For this review, take the finished solid that the model builds, in its own axes (mm). A direction names the side the tool comes from. Round coordinates to 2 decimals unless told otherwise and drop trailing zeros. Order: outer loops, then holes, each group sorted by start corner. A loop starts at its lowest first (then second) coordinate and runs counter-clockwise, first axis right, second up. Notation, with made-up numbers: (-20.5, -38) - (23.5, -38) arc R27 ccw to (23.5, -19) - close; hole circle Ø7 at (25, 51.25). An arc over 180 degrees is marked (long way). Write each question's results on one line, items separated by ' | '. Start each with the question number.
(1) For faces 1 (the flat face through (-19.35, -1.5, -6.77)), 2 (the flat face through (-20.227, -1.503, 43.929)), list the 3-axis set-ups (+Z, -Z, +X, -X, +Y, -Y) from which the entire face can be reached by the end or side of a thin tool; tool diameter is ignored.
(2) Take a section at B-B, the plane x = -4. Give the boundary of the cut face in (y, z), plus the area to 3 significant figures.
(3) For L1, parallel to X at y = -0.75, z = -46; L2, parallel to X at y = -2.05, z = 55.5; L3, parallel to X at y = -1.15, z = 69.5, list the stretches that pass through material, from the lowest coordinate up. Write a range as from..to.
(4) Take a section at A-A, the plane y = -1. Give the number of separate pieces and of enclosed holes in the cut face, plus the area to 3 significant figures.
(5) Take a section at C-C, the plane z = 37. Give the boundary of the cut face in (x, y).
(6) Draft analysis for pull direction Z (two halves, no side actions). For faces 3 (the flat face through (-45.517, -1.503, -15.58)), 4 (the flat face through (-30, 0, -3)), 5 (the cylindrical face through (-35.836, -1.503, -48.481)), state which applies: pulls with the +Z half, pulls with the -Z half, needs draft (parallel to the pull), parting line crosses it, or undercut.
(7) Insertion check: pin 1 Ø10 at (x, z) = (-38, 17) entering from +Y; pin 2 Ø1.5 at (y, z) = (-1.5, 2) entering from -X; pin 3 Ø6 at (x, z) = (-32.87, 17.29) entering from -Y. Each pin has a flat end and moves straight along its axis. Give the tip position at first contact, or say it passes through.
```python
from build123d import *

# Parameters (mm, degrees)
F0_R     = 3.175
F0_R_2   = 2.8967213822
F0_R_3   = 4.9231792558
F0_R_4   = 3.7359067091
F0_R_5   = 3.1164885501
F1_DEPTH = 3.048


with BuildPart() as f1:
    # F0 (on Front) → F1 (new body)
    with BuildSketch(Plane.XZ):
        with BuildLine():
            ThreePointArc((-42.3213338093, 69.2824711493), (-33.4675240871, 58.5855412551), (-23.3460408451, 68.0918461493))
            ThreePointArc((-23.3460408451, 68.0918461493), (-23.3647359509, 68.6883293913), (-23.4207478809, 69.2824711493))
            ThreePointArc((-23.4207478809, 69.2824711493), (-32.8710408451, 77.6168461493), (-42.3213338093, 69.2824711493))
        make_face()
        with Locations((-32.8710408451, 68.0918461493)):
            Circle(F0_R, mode=Mode.SUBTRACT)
        with BuildLine():
            ThreePointArc((-23.4207478809, 69.2824711493), (-23.3647359509, 68.6883293913), (-23.3460408451, 68.0918461493))
            ThreePointArc((-23.3460408451, 68.0918461493), (-33.4675240871, 58.5855412551), (-42.3213338093, 69.2824711493))
            Line((-42.3213338093, 69.2824711493), (-48.6215291188, 19.2762211493))
            ThreePointArc((-48.6215291188, 19.2762211493), (-32.8710408451, 33.1668461493), (-17.1205525714, 19.2762211493))
            Line((-17.1205525714, 19.2762211493), (-23.4207478809, 69.2824711493))
        make_face()
        with Locations((-36.0460408451, 53.8170461493)):
            Circle(F0_R_2, mode=Mode.SUBTRACT)
        with BuildLine():
            ThreePointArc((-16.9960408451, 17.2918461493), (-17.0271993547, 18.2859848859), (-17.1205525714, 19.2762211493))
            ThreePointArc((-17.1205525714, 19.2762211493), (-32.8710408451, 33.1668461493), (-48.6215291188, 19.2762211493))
            ThreePointArc((-48.6215291188, 19.2762211493), (-48.7457796213, 17.2007759138), (-48.5977252432, 15.1268928374))
            ThreePointArc((-48.5977252432, 15.1268928374), (-32.5863651682, 1.4193988031), (-17.0768380415, 15.6922265698))
            ThreePointArc((-17.0768380415, 15.6922265698), (-17.0162530114, 16.4910167377), (-16.9960408451, 17.2918461493))
        make_face()
        with Locations((-32.8710408451, 17.2918461493)):
            Circle(F0_R_3, mode=Mode.SUBTRACT)
        with BuildLine():
            ThreePointArc((-17.0768380415, 15.6922265698), (-32.5863651682, 1.4193988031), (-48.5977252432, 15.1268928374))
            Line((-48.5977252432, 15.1268928374), (-42.3484581137, -47.1590412869))
            ThreePointArc((-42.3484581137, -47.1590412869), (-39.8191713507, -39.692855893), (-32.5308622319, -36.6892304078))
            Line((-32.5308622319, -36.6892304078), (-22.4185752351, -37.0506140669))
            Line((-22.4185752351, -37.0506140669), (-21.5634638108, -28.6074795691))
            Line((-21.5634638108, -28.6074795691), (-17.0768380415, 15.6922265698))
        make_face()
        with BuildLine():
            ThreePointArc((-32.5308622319, -36.6892304078), (-39.8191713507, -39.692855893), (-42.3484581137, -47.1590412869))
            ThreePointArc((-42.3484581137, -47.1590412869), (-39.1340347775, -53.3845409642), (-32.5308622705, -55.727077295))
            ThreePointArc((-32.5308622705, -55.727077295), (-26.0166325584, -52.8219811873), (-23.3460408451, -46.2081538507))
            ThreePointArc((-23.3460408451, -46.2081538507), (-26.0166325449, -39.594326528), (-32.5308622319, -36.6892304078))
        make_face()
        with Locations((-32.8710408451, -46.2081538507)):
            Circle(F0_R_4, mode=Mode.SUBTRACT)
        with BuildLine():
            Line((-22.4185752351, -37.0506140669), (-32.5308622319, -36.6892304078))
            ThreePointArc((-32.5308622319, -36.6892304078), (-26.0166325449, -39.594326528), (-23.3460408451, -46.2081538507))
            Line((-23.3460408451, -46.2081538507), (-22.4185752351, -37.0506140669))
        make_face()
        with BuildLine():
            ThreePointArc((-13.9376627644, -37.3536971559), (-19.6460678, -34.6332730975), (-21.5634638108, -28.6074795691))
            Line((-21.5634638108, -28.6074795691), (-22.4185752351, -37.0506140669))
            Line((-22.4185752351, -37.0506140669), (-13.9376627644, -37.3536971559))
        make_face()
        with BuildLine():
            ThreePointArc((-23.3460408451, -46.2081538507), (-26.0166325584, -52.8219811873), (-32.5308622705, -55.727077295))
            Line((-32.53086227, -55.7270773096), (11.8624413004, -54.1405900542))
            ThreePointArc((11.8624413004, -54.1405900542), (3.6414591549, -46.2081538504), (11.862441301, -38.2757176472))
            Line((11.8624413004, -38.2757176655), (-13.9376627644, -37.3536971559))
            Line((-13.9376627644, -37.3536971559), (-22.4185752351, -37.0506140669))
            Line((-22.4185752351, -37.0506140669), (-23.3460408451, -46.2081538507))
        make_face()
        with BuildLine():
            ThreePointArc((11.862441301, -38.2757176472), (3.6414591549, -46.2081538504), (11.8624413004, -54.1405900542))
            ThreePointArc((11.8624413004, -54.1405900542), (17.2909660605, -51.7196766312), (19.5164591549, -46.2081538507))
            ThreePointArc((19.5164591549, -46.2081538507), (17.2909660607, -40.6966310704), (11.862441301, -38.2757176472))
        make_face()
        with Locations((11.5789591549, -46.2081538507)):
            Circle(F0_R_5, mode=Mode.SUBTRACT)
    extrude(amount=F1_DEPTH)


solid = f1.part
```
Results below:
1) face 1: +X, +Y, -Y | face 2: +Z, +X, +Y, -Y
2) outline: (-3.05, -54.71) - (0, -54.71) - (0, -37.71) - (-3.05, -37.71) - close | area: 51.8 mm^2
3) L1: x = -42.46..-36.6, -29.14..8.47, 14.69..19.51 | L2: x = -44.06..-38.4, -33.69..-21.68 | L3: x = -42.29..-35.72, -30.03..-23.45
4) separate pieces: 1 | enclosed holes: 5 | area: 3,720 mm^2
5) outline: (-46.39, -3.05) - (-19.35, -3.05) - (-19.35, 0) - (-46.39, 0) - close
6) face 3: pulls with the -Z half | face 4: needs draft | face 5: undercut
7) pin 1: stops at y = 0 | pin 2: stops at x = -47.36 | pin 3: passes through
